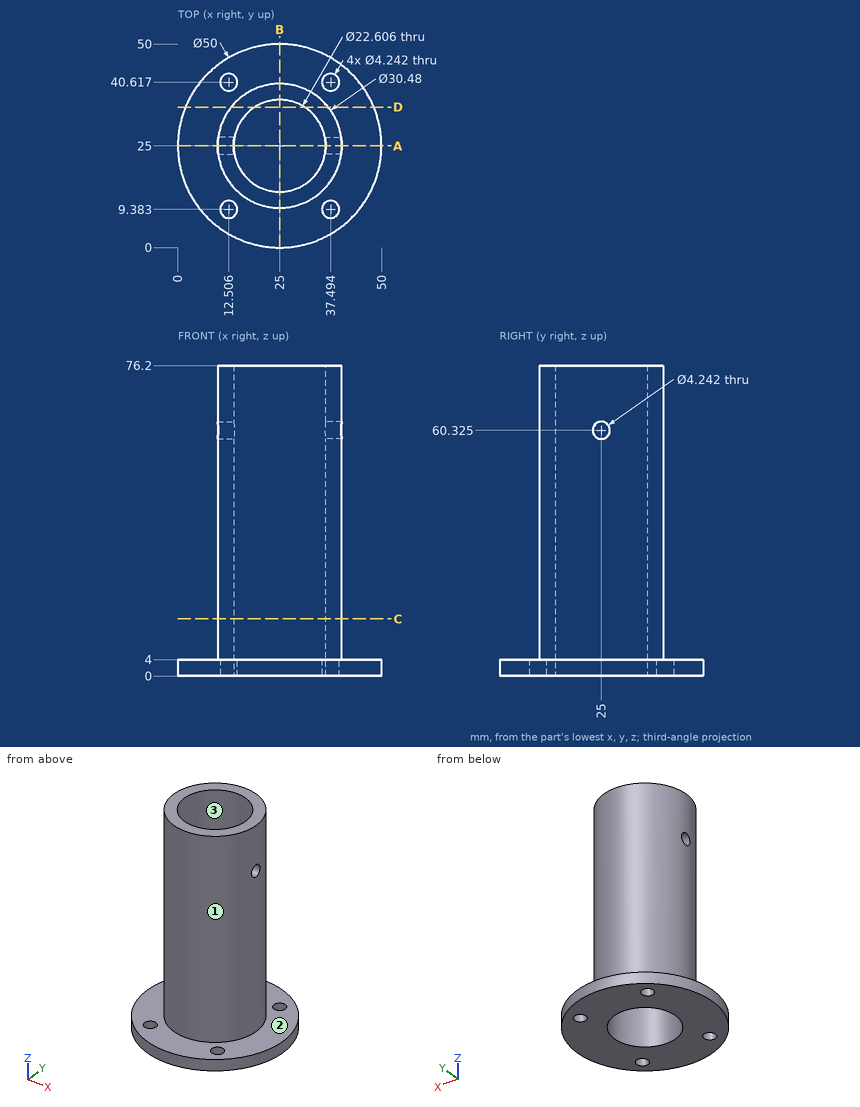
Here's the drawing with two shaded views (mm, measured from the low corner). I have some questions. Coordinates: 2 decimals unless noted, no trailing zeros. Order: outer loops, then holes, each group sorted by start corner. A loop starts at its lowest first (then second) coordinate and runs counter-clockwise, first axis right, second up.
Item 1: I need wall thicknesses on line 1 (X direction, y = 25, z = 49); line 2 (Z direction, x = 17.5, y = 42); line 3 (X direction, y = 19, z = 6). Which ranges of each line are inside material? Lowest first, please.
Result sheet:
line 1: x = 9.76 to 13.7, 36.3 to 40.24
line 2: z = 0 to 4
line 3: x = 10.99 to 15.42, 34.58 to 39.01
Item 2: If we section it at B-B on x = 25: List the corners of the cut face in (y, z) for me.
Result sheet:
outline: (0, 0) - (13.7, 0) - (13.7, 76.2) - (9.76, 76.2) - (9.76, 4) - (0, 4) - close; (36.3, 0) - (50, 0) - (50, 4) - (40.24, 4) - (40.24, 76.2) - (36.3, 76.2) - close
Item 3: If we mould it in two halves opening along X, with no side actions, what happens to the marked faces 1, 2 and 3? For each: +X half, -X half, draft (parallel to the pull), parting line (faces both ways), or undercut.
Result sheet:
face 1: parting line
face 2: draft
face 3: undercut
Item 4: If we section it at A-A on y = 25: List the corners of the cut face in (x, z) for me.
Result sheet:
outline: (0, 0) - (13.7, 0) - (13.7, 58.2) - (9.76, 58.2) - (9.76, 4) - (0, 4) - close; (9.76, 62.45) - (13.7, 62.45) - (13.7, 76.2) - (9.76, 76.2) - close; (36.3, 0) - (50, 0) - (50, 4) - (40.24, 4) - (40.24, 58.2) - (36.3, 58.2) - close; (36.3, 62.45) - (40.24, 62.45) - (40.24, 76.2) - (36.3, 76.2) - close
Item 5: If we section it at C-C on z = 14: List the corners of the cut face in (x, y) for me.
Result sheet:
outline: circle Ø30.48 at (25, 25); hole circle Ø22.61 at (25, 25)
Item 6: For P1, Ø5, axis at y = 25, z = 60.325, coming from the +X side; P2, Ø5.5, axis at x = 37.49, y = 9.38, coming from the +Z side; P3, Ø2.5, axis at x = 12.51, y = 9.38, coming from the +Z side; P4, Ø5, axis at y = 16.5, z = 40.5, coming from the -X side, each with a flat end and sliding along its axis, tell me the tip position at first contact or that it passes through.
Result sheet:
P1: stops at x = 40.24
P2: stops at z = 4
P3: passes through
P4: stops at x = 10.99
Item 7: If we section it at D-D on y = 34.5: List the corners of the cut face in (x, z) for me (1 decimal).
Result sheet:
outline: (1.9, 0) - (18.9, 0) - (18.9, 76.2) - (13.1, 76.2) - (13.1, 4) - (1.9, 4) - close; (31.1, 0) - (48.1, 0) - (48.1, 4) - (36.9, 4) - (36.9, 76.2) - (31.1, 76.2) - close
